```python
from build123d import *

# Parameters (mm, degrees)
SKETCH1_W           = 52.5
SKETCH1_H           = 36.5
SKETCH1_R           = 1.5
BOSS_EXTRUDE1_DEPTH = 1.5
SKETCH2_W           = 16
SKETCH2_H           = 11.5
BOSS_EXTRUDE2_DEPTH = 10.5
SKETCH7_W           = 5
SKETCH7_H           = 3
CUT_EXTRUDE1_DEPTH  = 10


with BuildPart() as part:
    # Sketch1 → Boss-Extrude1 (new body)
    with BuildSketch(Plane(origin=(0, 0, 0), x_dir=(1, 0, 0), z_dir=(0, 1, 0))):
        Rectangle(SKETCH1_W, SKETCH1_H)
        with Locations((-23.25, 15.25)):
            Circle(SKETCH1_R, mode=Mode.SUBTRACT)
        with Locations((23.25, 15.25)):
            Circle(SKETCH1_R, mode=Mode.SUBTRACT)
        with Locations((-23.25, -15.25)):
            Circle(SKETCH1_R, mode=Mode.SUBTRACT)
        with Locations((23.25, -15.25)):
            Circle(SKETCH1_R, mode=Mode.SUBTRACT)
    extrude(amount=BOSS_EXTRUDE1_DEPTH)

    # Sketch2 → Boss-Extrude2 (add)
    with BuildSketch(Plane(origin=(0, 1.5, 0), x_dir=(1, 0, 0), z_dir=(0, 1, 0))):
        with Locations((24.75, 0)):
            Rectangle(SKETCH2_W, SKETCH2_H)
    extrude(amount=BOSS_EXTRUDE2_DEPTH)

    # Sketch7 → Cut-Extrude1 (cut)
    with BuildSketch(Plane(origin=(32.75, 0, 0), x_dir=(0, 0, -1), z_dir=(1, 0, 0))):
        Polygon((-4.75, 2.5), (4.75, 2.5), (4.75, 9), (2.75, 11), (-2.75, 11), (-4.75, 9), align=None)
        with Locations((0, 6.75)):
            Rectangle(SKETCH7_W, SKETCH7_H, mode=Mode.SUBTRACT)
    extrude(amount=-CUT_EXTRUDE1_DEPTH, mode=Mode.SUBTRACT)


solid = part.part
```
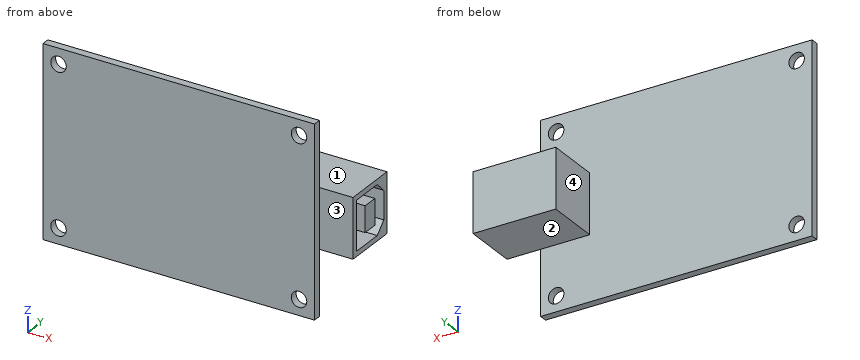
Source: CAD feature listing. Evaluate the final solid. Frame: model axes, mm. Face numbers are marked on the shaded views. A direction names the side the tool comes from. Round coordinates to 2 decimals unless told otherwise and drop trailing zeros. Loops run counter-clockwise (first coordinate to the right, second up) from the corner with the lowest first, then second, coordinate; pieces in that order, holes last. Notation, with made-up numbers: M 73,39 L 80,39 A10 ccw 80,54 Z; hole C -27,72 d4. An arc over 180 degrees is marked long. Use a Markdown table: item, result. Add a question column.
1. Ray query, line 1 along X through (y, z) = (0.8, 15.25); line 2 along Z through (x, y) = (23.25, 0.6); line 3 along Z through (x, y) = (28.5, 6.5). Return the intervals inside material, ascending. Write a range as [from, to].
2. Cut plane D-D, the plane z = 10. Output: boundary loops of the cut face in (x, y), and give its area (4 significant figures).
3. Contact query for flat-ended pins moving along their axis: pin 1 (1.6 mm diameter, centred on x = 26, z = -1.5, fed in from -Y); pin 2 (3 mm diameter, centred on x = 28, y = 4.5, fed in from -Z); pin 3 (0.9 mm diameter, centred on x = 28.5, y = 7, fed in from +Z); pin 4 (2.5 mm diameter, centred on x = 30, z = -1, fed in from -Y). Output: stop coordinate, or through.
4. Set-up query: the marked faces 1, 2, 3 and 4. Return all of +Z, -Z, +X, -X, +Y, -Y with unobstructed straight access to the full face (end or side cutting, diameter ignored); none if empty.
5. Cut plane B-B, the plane z = -15.25. Output: boundary loops of the cut face in (x, y).
6. Cut plane A-A, the plane x = -23.25. Output: boundary loops of the cut face in (y, z).
7. Cut plane C-C, the plane y = 4.5. Output: boundary loops of the cut face in (x, z).
Solution:
| question | item | result |
|---|---|---|
| 1 | line 1 | x = [-26.25, -24.75], [-21.75, 21.75], [24.75, 26.25] |
| 1 | line 2 | z = [-18.25, -16.75], [-13.75, 13.75], [16.75, 18.25] |
| 1 | line 3 | z = [-5.75, -4.75], [-2.5, 2.5], [4.75, 5.75] |
| 2 | outline | M -26.25,0 L 26.25,0 L 26.25,1.5 L -26.25,1.5 Z |
| 2 | area | 78.75 mm2 |
| 3 | pin 1 | stops at y = 0 |
| 3 | pin 2 | stops at z = -5.75 |
| 3 | pin 3 | stops at z = 5.75 |
| 3 | pin 4 | stops at y = 1.5 |
| 4 | face 1 | +Z, +X, -X, +Y |
| 4 | face 2 | -Z, +X, -X, +Y |
| 4 | face 3 | +Z, -Z, +X, -Y |
| 4 | face 4 | +Z, -Z, -X, +Y |
| 5 | outline | M -26.25,0 L -24.75,0 L -24.75,1.5 L -26.25,1.5 Z; M -21.75,0 L 21.75,0 L 21.75,1.5 L -21.75,1.5 Z; M 24.75,0 L 26.25,0 L 26.25,1.5 L 24.75,1.5 Z |
| 6 | outline | M 0,-18.25 L 1.5,-18.25 L 1.5,-16.75 L 0,-16.75 Z; M 0,-13.75 L 1.5,-13.75 L 1.5,13.75 L 0,13.75 Z; M 0,16.75 L 1.5,16.75 L 1.5,18.25 L 0,18.25 Z |
| 7 | outline | M 16.75,-5.75 L 32.75,-5.75 L 32.75,-4.75 L 22.75,-4.75 L 22.75,4.75 L 32.75,4.75 L 32.75,5.75 L 16.75,5.75 Z |
